Source: CAD feature listing. Evaluate the final solid. Frame: model axes, mm. Coordinates: 2 decimals unless noted, no trailing zeros. Write each loop counter-clockwise with the first axis right and the second up, starting at its lowest first coordinate (ties: lowest second). Pieces come first, ordered by that corner, then holes. Notation, with made-up numbers: (-25.75, 38) - (22.25, 38) arc R17 ccw to (22.25, 54) - close; hole circle Ø4 at (63.25, 37.5). An arc over 180 degrees is marked (long way). One line per question, with ' | ' between items.
from build123d import *

# Parameters (mm, degrees)
F1_DEPTH = 5.55625
F2_R     = 3.175
F3_DEPTH = 5.55625


with BuildPart() as f1:
    # F0 (on Top) → F1 (new body)
    with BuildSketch(Plane.XY):
        Polygon((-0.346295, -6.406452), (5.375003, -3.503126), (5.721298, 2.903326), (0.346295, 6.406452), (-5.375003, 3.503126), (-5.721298, -2.903326), align=None)
    extrude(amount=-F1_DEPTH)

    # F2 (on face) → F3 (cut, through all)
    with BuildSketch(Plane.XY):
        Circle(F2_R)
    extrude(amount=-F3_DEPTH, mode=Mode.SUBTRACT)


solid = f1.part
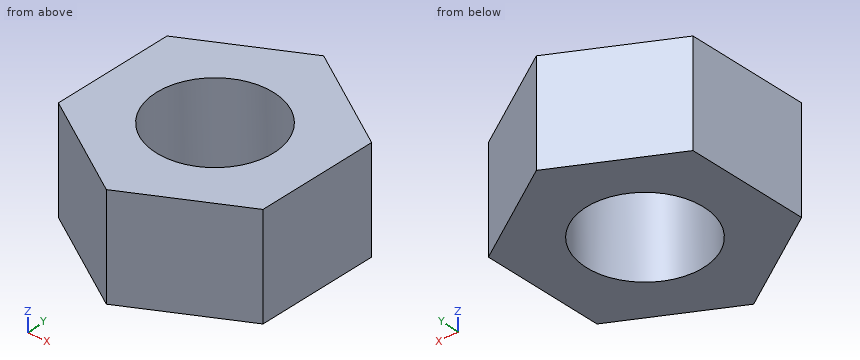
Item 1: Cut plane B-B on z = -1.15. Return loops of the section in (x, y) (3 decimals).
Check sheet entries:
outline: (-5.721, -2.903) - (-0.346, -6.406) - (5.375, -3.503) - (5.721, 2.903) - (0.346, 6.406) - (-5.375, 3.503) - close; hole circle Ø6.35 at (0, 0)
Item 2: Cut plane D-D on x = 4.5. Return loops of the section in (y, z), and give its area (3 significant figures).
Check sheet entries:
outline: (-3.95, -5.56) - (3.7, -5.56) - (3.7, 0) - (-3.95, 0) - close | area: 42.5 mm²
Item 3: Cut plane C-C on x = 1.5. Return loops of the section in (y, z).
Check sheet entries:
outline: (-5.47, -5.56) - (-2.8, -5.56) - (-2.8, 0) - (-5.47, 0) - close; (2.8, -5.56) - (5.65, -5.56) - (5.65, 0) - (2.8, 0) - close
Item 4: Cut plane A-A on y = 0. Return loops of the section in (x, z) (3 decimals), and give its area (3 significant figures).
Check sheet entries:
outline: (-5.564, -5.556) - (-3.175, -5.556) - (-3.175, 0) - (-5.564, 0) - close; (3.175, -5.556) - (5.564, -5.556) - (5.564, 0) - (3.175, 0) - close | area: 26.6 mm²
Item 5: Pin query (flat end, axial travel): pin 1 Ø1.5 at (y, z) = (-3, -2) entering from +X; pin 2 Ø3 at (x, z) = (0.5, -2.5) entering from +Y; pin 3 Ø1 at (x, z) = (-3, -4) entering from +Y; pin 4 Ø1 at (x, z) = (-0.5, -2.5) entering from +Y. Return the tip coordinate at first contact, or that it passes through.
Check sheet entries:
pin 1: x = 5.44 | pin 2: y = 6.41 | pin 3: y = 4.96 | pin 4: y = 6.23
Item 6: Ray query, line 1 along Y through (x, z) = (-0.25, -1.25); line 2 along Y through (x, z) = (0, -4) (3 decimals); line 3 along X through (y, z) = (-2.75, -1.95). Return the intervals inside material, ascending. Write a range as [from, to].
Check sheet entries:
line 1: [-6.36, -3.17], [3.17, 6.1] | line 2: [-6.231, -3.175], [3.175, 6.231] | line 3: [-5.71, -1.59], [1.59, 5.42]
